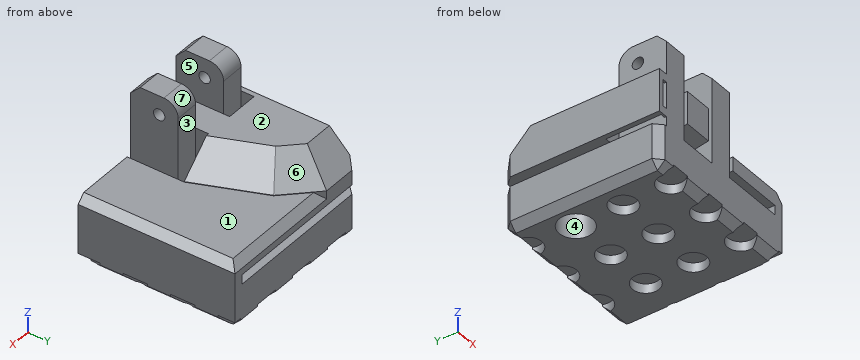
from build123d import *

# Parameters (mm, degrees)
SKETCH_W             = 35
SKETCH_H             = 33
PAD_DEPTH            = 20
SKETCH001_W          = 7
SKETCH001_H          = 12
POCKET_DEPTH         = 10
SKETCH004_W          = 36
SKETCH004_H          = 2
POCKET002_DEPTH      = 18.001
POCKET002_DEPTH_BACK = 15.001
SKETCH002_W          = 5
SKETCH002_H          = 10
PAD001_DEPTH         = 20
SKETCH003_R          = 1.2
POCKET001_DEPTH      = 22.001
POCKET003_DEPTH      = 6
CHAMFER_SIZE         = 5.9
CHAMFER001_SIZE      = 1.6
CHAMFER002_SIZE      = 2
FILLET_R             = 3
SKETCH010_R          = 2.8
POCKET006_DEPTH      = 2
LINEARPATTERN_COUNT  = 4
LINEARPATTERN_PITCH  = 10
SKETCH012_R          = 3.5
POCKET007_DEPTH      = 8
SKETCH013_W          = 3.523392
SKETCH013_H          = 1.7
SKETCH013_W_2        = 3.89822
PAD003_DEPTH         = 0.4
POCKET008_DEPTH      = 6


with BuildPart() as part:
    # Sketch → Pad (new body)
    with BuildSketch(Plane.XY):
        with Locations((-4.5, 1.5)):
            Rectangle(SKETCH_W, SKETCH_H)
    extrude(amount=PAD_DEPTH)

    # Sketch001 (on Face6 of Pad) → Pocket (cut)
    with BuildSketch(Plane.XY.offset(20)):
        with Locations((-17.5, -9)):
            Rectangle(SKETCH001_W, SKETCH001_H)
        with Locations((-4.5, -9)):
            Rectangle(SKETCH001_W, SKETCH001_H)
    extrude(amount=-POCKET_DEPTH, mode=Mode.SUBTRACT)

    # Sketch004 → Pocket002 (cut, two sides)
    with BuildSketch(Plane.XZ) as pocket002_sk:
        with Locations((-7, 10)):
            Rectangle(SKETCH004_W, SKETCH004_H)
    extrude(amount=-POCKET002_DEPTH, mode=Mode.SUBTRACT)
    extrude(pocket002_sk.sketch, amount=POCKET002_DEPTH_BACK, mode=Mode.SUBTRACT)

    # Sketch002 (on Face8 of Pocket002) → Pad001 (join)
    with BuildSketch(Plane.XY.offset(9)):
        with Locations((-17.5, -10)):
            Rectangle(SKETCH002_W, SKETCH002_H)
        with Locations((-4.5, -10)):
            Rectangle(SKETCH002_W, SKETCH002_H)
    extrude(amount=PAD001_DEPTH)

    # Sketch003 → Pocket001 (cut, through all)
    with BuildSketch(Plane.YZ):
        with Locations((-9, 25)):
            Circle(SKETCH003_R)
    extrude(amount=-POCKET001_DEPTH, mode=Mode.SUBTRACT)

    # Sketch005 (on Face4 of Pocket001) → Pocket003 (cut)
    with BuildSketch(Plane.XY.offset(20)):
        Polygon((-6.878414, 11.506697), (-1, -3), (-1, -16.521692), (16.145611, -16.521692), (16.145611, 20.333527), (-18.556482, 20.333527), (-13.204168, 18), align=None)
    extrude(amount=-POCKET003_DEPTH, mode=Mode.SUBTRACT)

    # Chamfer
    chamfer_edges = [part.edges().sort_by_distance(p)[0] for p in [
        (-17.602084, 18, 20),
        (-10.041291, 14.753349, 20),
        (-3.939207, 4.253349, 20),
    ]]
    chamfer(chamfer_edges, length=CHAMFER_SIZE)

    # Chamfer001
    chamfer001_edges = [part.edges().sort_by_distance(p)[0] for p in [
        (-4.5, 18, 0),
        (13, 1.5, 0),
        (-4.5, -15, 0),
        (-22, 1.5, 0),
        (-22, 18, 4.5),
        (-22, -15, 4.5),
        (-22, 18, 12.55),
        (13, 1.5, 14),
        (-0.102084, 18, 14),
    ]]
    chamfer(chamfer001_edges, length=CHAMFER001_SIZE)

    # Chamfer002
    chamfer002_edges = [part.edges().sort_by_distance(p)[0] for p in [
        (-17.5, -15, 29),
        (-4.5, -15, 29),
    ]]
    chamfer(chamfer002_edges, length=CHAMFER002_SIZE)

    # Fillet
    fillet_edges = [part.edges().sort_by_distance(p)[0] for p in [
        (-4.5, -5, 29),
        (-17.5, -5, 29),
    ]]
    fillet(fillet_edges, radius=FILLET_R)

    # Sketch010 → Pocket006 (cut)
    with BuildSketch(Plane.XY):
        with Locations((14, -13)):
            Circle(SKETCH010_R)
        with Locations((4, -13)):
            Circle(SKETCH010_R)
        with Locations((-6, -13)):
            Circle(SKETCH010_R)
        with Locations((-16, -13)):
            Circle(SKETCH010_R)
    pocket006 = extrude(amount=POCKET006_DEPTH, mode=Mode.SUBTRACT)

    # LinearPattern: Pocket006 ×4
    with Locations(*[(0, i * LINEARPATTERN_PITCH, 0) for i in range(1, LINEARPATTERN_COUNT)]):
        add(pocket006, mode=Mode.SUBTRACT)

    # Sketch012 (on Face5 of Pad) → Pocket007 (cut)
    with BuildSketch(Plane(origin=(0, 0, 0), x_dir=(1, 0, 0), z_dir=(0, 0, -1))):
        with Locations((-16, -7)):
            Circle(SKETCH012_R)
    extrude(amount=-POCKET007_DEPTH, mode=Mode.SUBTRACT)

    # Sketch013 (on Face3 of Pad) → Pad003 (join)
    with BuildSketch(Plane.XZ.offset(15)):
        with Locations((-19.82605, 19.15)):
            Rectangle(SKETCH013_W, SKETCH013_H)
        with Locations((-19.451214, 11.85)):
            Rectangle(SKETCH013_W_2, SKETCH013_H)
    extrude(amount=-PAD003_DEPTH)

    # Sketch014 (on Face9 of Pocket) → Pocket008 (cut)
    with BuildSketch(Plane(origin=(-14, 0, 0), x_dir=(0, -1, 0), z_dir=(-1, 0, 0))):
        Polygon((3, 11), (23, 14.52654), (23, 11), align=None)
    extrude(amount=-POCKET008_DEPTH, mode=Mode.SUBTRACT)


solid = part.part
Work out the finished part from the listing and answer in its coordinate system (mm). Face numbers are marked on the shaded views. A direction names the side the tool comes from. Round coordinates to 2 decimals unless told otherwise and drop trailing zeros. Loops run counter-clockwise (first coordinate to the right, second up) from the corner with the lowest first, then second, coordinate; pieces in that order, holes last. Notation, with made-up numbers: (-12, 4.25) - (43, 4.25) arc R21 ccw to (43, 23.25) - close; hole circle Ø10 at (43.25, -35). An arc over 180 degrees is marked (long way). One line per item, written item: value.
Q1. Find section B-B on z = 3.5. Give the vertices of the cut face in (x, y).
Check values:
outline: (-22, -13.4) - (-20.4, -15) - (13, -15) - (13, 18) - (-20.4, 18) - (-22, 16.4) - close; hole circle Ø7 at (-16, 7)
Q2. Find section D-D on z = 25. Give the vertices of the cut face in (x, y), and give its area (3 significant figures).
Check values:
outline: (-20, -15) - (-15, -15) - (-15, -10.2) - (-20, -10.2) - close; (-20, -7.8) - (-15, -7.8) - (-15, -5) - (-20, -5) - close; (-7, -15) - (-2, -15) - (-2, -10.2) - (-7, -10.2) - close; (-7, -7.8) - (-2, -7.8) - (-2, -5) - (-7, -5) - close
area: 76.0 mm2
Q3. Find section A-A on x = -6. Give the vertices of the cut face in (y, z).
Check values:
outline: (-15, 2) - (-10.2, 2) - (-10.2, 0) - (-5.8, 0) - (-5.8, 2) - (-0.2, 2) - (-0.2, 0) - (4.2, 0) - (4.2, 2) - (9.8, 2) - (9.8, 0) - (14.2, 0) - (14.2, 2) - (18, 2) - (18, 9) - (-5, 9) - (-5, 26) arc R3 ccw to (-8, 29) - (-13, 29) - (-15, 27) - close; (-3, 11) - (18, 11) - (18, 12.4) - (16.4, 14) - (9.34, 14) - (9.34, 14.1) - (-3, 18.73) - close; hole circle Ø2.4 at (-9, 25)
Q4. Each of these flat-tipped pins is pushed along its axis until it touches: pin 1 Ø1.9 at (x, y) = (3, 15.5) entering from -Z; pin 2 Ø4.5 at (x, y) = (-11.5, -4) entering from +Z; pin 3 Ø2 at (x, y) = (7, -4) entering from +Z; pin 4 Ø6 at (x, y) = (4.5, -2.5) entering from -Z. Where does it stop, or does it pass through?
Check values:
pin 1: z = 2
pin 2: z = 20
pin 3: z = 14
pin 4: z = 0
Q5. Find section C-C on x = 4. Give the vertices of the cut face in (y, z).
Check values:
outline: (-15, 2) - (-10.2, 2) - (-10.2, 0) - (-5.8, 0) - (-5.8, 2) - (-0.2, 2) - (-0.2, 0) - (4.2, 0) - (4.2, 2) - (9.8, 2) - (9.8, 0) - (14.2, 0) - (14.2, 2) - (18, 2) - (18, 9) - (-15, 9) - close; (-15, 11) - (18, 11) - (18, 12.4) - (16.4, 14) - (-15, 14) - close
Q6. For the marked faces 1, 2, 3 and 4, determine the directions among +Z, -Z, +X, -X, +Y, -Y from which every point of the face is accessible in a straight line to the end or side of a thin tool.
Check values:
face 1: +Z, +X, +Y
face 2: +Z, +Y
face 3: +Z
face 4: -Z
Q7. Straight lines are drawn through the part: probe 1 along Y at (x, z) = (4, 0.55); probe 2 along X at (y, z) = (-7.5, 15); probe 3 along Y at (x, z) = (-16, 1.45). For each, find the intervals that lie inside material, in ascending order.
Check values:
probe 1: -10.2 to -5.8, -0.2 to 4.2, 9.8 to 14.2
probe 2: -22 to -21, -20 to -15, -14 to -8, -7 to -2
probe 3: -10.2 to -5.8, -0.2 to 3.5, 10.5 to 14.2
Q8. The mould has two halves that part along X. Classify the marked faces 5, 6 and 7: +X half, -X half, draft (parallel to the pull), parting line (faces both ways), or undercut.
Check values:
face 5: undercut
face 6: +X half
face 7: draft
